```python
from build123d import *

# Parameters (mm, degrees)
SKETCH2_W               = 150
SKETCH2_H               = 180
BOSS_EXTRUDE1_DEPTH     = 4
SKETCH3_R               = 2
SKETCH3_W               = 23
SKETCH3_H               = 42
CUT_EXTRUDE1_DEPTH      = 118.426572802
MIRROR2_COPY_1_SKETCH_R = 2
MIRROR2_COPY_1_SKETCH_W = 23
MIRROR2_COPY_1_SKETCH_H = 42
MIRROR2_COPY_1_DEPTH    = 118.426572802
FILLET1_SIZE            = 10
FILLET1_SIZE_2          = 20
FILLET2_SIZE            = 10
FILLET2_SIZE_2          = 20
SKETCH4_W               = 50
SKETCH4_H               = 100
CUT_EXTRUDE2_DEPTH      = 118.426572949
SKETCH5_R               = 2.5
CUT_EXTRUDE3_DEPTH      = 118.426572949
SKETCH6_R               = 2.5
CUT_EXTRUDE4_DEPTH      = 118.426572949


with BuildPart() as part:
    # Sketch2 → Boss-Extrude1 (new, symmetric)
    with BuildSketch(Plane(origin=(0, 0, 0), x_dir=(1, 0, 0), z_dir=(0, 1, 0))):
        Rectangle(SKETCH2_W, SKETCH2_H)
    extrude(amount=BOSS_EXTRUDE1_DEPTH, both=True)

    # Sketch3 → Cut-Extrude1 (cut, through all)
    with BuildSketch(Plane(origin=(0, 4, 0), x_dir=(1, 0, 0), z_dir=(0, 1, 0))):
        with Locations(Location((-59.95, -34.7, 0), (0, 0, 270))):
            Circle(SKETCH3_R)
        with Locations(Location((-50.05, -34.7, 0), (0, 0, 270))):
            Circle(SKETCH3_R)
        with Locations(Location((-59.95, -83.3, 0), (0, 0, 270))):
            Circle(SKETCH3_R)
        with Locations(Location((-50.05, -83.3, 0), (0, 0, 270))):
            Circle(SKETCH3_R)
        with Locations((-55, -59)):
            Rectangle(SKETCH3_W, SKETCH3_H)
    cut_extrude1 = extrude(amount=-CUT_EXTRUDE1_DEPTH, mode=Mode.SUBTRACT)

    # Mirror1: Cut-Extrude1 across plane
    add(cut_extrude1.mirror(Plane.XY), mode=Mode.SUBTRACT)

    # Mirror2: Cut-Extrude1 across plane
    add(cut_extrude1.mirror(Plane(origin=(0, 0, 0), x_dir=(0, 0, 1), z_dir=(1, 0, 0))), mode=Mode.SUBTRACT)

    # Mirror2 copy 1 sketch → Mirror2 copy 1 (cut, through all)
    with BuildSketch(Plane(origin=(0, 4, 0), x_dir=(-1, 0, 0), z_dir=(0, 1, 0))):
        with Locations(Location((-59.95, -34.7, 0), (0, 0, 270))):
            Circle(MIRROR2_COPY_1_SKETCH_R)
        with Locations(Location((-50.05, -34.7, 0), (0, 0, 270))):
            Circle(MIRROR2_COPY_1_SKETCH_R)
        with Locations(Location((-59.95, -83.3, 0), (0, 0, 270))):
            Circle(MIRROR2_COPY_1_SKETCH_R)
        with Locations(Location((-50.05, -83.3, 0), (0, 0, 270))):
            Circle(MIRROR2_COPY_1_SKETCH_R)
        with Locations((-55, -59)):
            Rectangle(MIRROR2_COPY_1_SKETCH_W, MIRROR2_COPY_1_SKETCH_H)
    extrude(amount=-MIRROR2_COPY_1_DEPTH, mode=Mode.SUBTRACT)

    # Fillet1
    # an asymmetric fillet: 20, 10 mm, written as the material it takes off along each edge
    with BuildSketch(Plane(origin=(-75, -54, -90), x_dir=(1, 0, 0), z_dir=(0, 1, 0))) as fillet1_piece_1:
        with BuildLine():
            Bezier((FILLET1_SIZE, 0), (0, 0), (0, -FILLET1_SIZE_2), weights=[1, 0.707106781, 1])
            Line((0, -FILLET1_SIZE_2), (0, 0))
            Line((0, 0), (FILLET1_SIZE, 0))
        make_face()
    extrude(amount=108, mode=Mode.SUBTRACT)
    with BuildSketch(Plane(origin=(75, 54, 90), x_dir=(0, 0, -1), z_dir=(0, -1, 0))) as fillet1_piece_2:
        with BuildLine():
            Bezier((FILLET1_SIZE_2, 0), (0, 0), (0, -FILLET1_SIZE), weights=[1, 0.707106781, 1])
            Line((0, -FILLET1_SIZE), (0, 0))
            Line((0, 0), (FILLET1_SIZE_2, 0))
        make_face()
    extrude(amount=108, mode=Mode.SUBTRACT)

    # Fillet2
    # an asymmetric fillet: 20, 10 mm, written as the material it takes off along each edge
    with BuildSketch(Plane(origin=(75, 54, -90), x_dir=(-1, 0, 0), z_dir=(0, -1, 0))) as fillet2_piece_1:
        with BuildLine():
            Bezier((FILLET2_SIZE, 0), (0, 0), (0, -FILLET2_SIZE_2), weights=[1, 0.707106781, 1])
            Line((0, -FILLET2_SIZE_2), (0, 0))
            Line((0, 0), (FILLET2_SIZE, 0))
        make_face()
    extrude(amount=108, mode=Mode.SUBTRACT)
    with BuildSketch(Plane(origin=(-75, -54, 90), x_dir=(0, 0, -1), z_dir=(0, 1, 0))) as fillet2_piece_2:
        with BuildLine():
            Bezier((FILLET2_SIZE_2, 0), (0, 0), (0, -FILLET2_SIZE), weights=[1, 0.707106781, 1])
            Line((0, -FILLET2_SIZE), (0, 0))
            Line((0, 0), (FILLET2_SIZE_2, 0))
        make_face()
    extrude(amount=108, mode=Mode.SUBTRACT)

    # Sketch4 → Cut-Extrude2 (cut, through all)
    with BuildSketch(Plane(origin=(0, 4, 0), x_dir=(1, 0, 0), z_dir=(0, 1, 0))):
        Rectangle(SKETCH4_W, SKETCH4_H)
    extrude(amount=-CUT_EXTRUDE2_DEPTH, mode=Mode.SUBTRACT)

    # Sketch5 → Cut-Extrude3 (cut, through all)
    with BuildSketch(Plane(origin=(0, 4, 0), x_dir=(1, 0, 0), z_dir=(0, 1, 0))):
        with Locations(Location((-25, 81, 0), (0, 0, 270))):
            Circle(SKETCH5_R)
        with Locations(Location((25, 81, 0), (0, 0, 270))):
            Circle(SKETCH5_R)
        with Locations(Location((0, 81, 0), (0, 0, 270))):
            Circle(SKETCH5_R)
        with Locations(Location((-25, 70, 0), (0, 0, 270))):
            Circle(SKETCH5_R)
        with Locations(Location((0, 70, 0), (0, 0, 270))):
            Circle(SKETCH5_R)
        with Locations(Location((25, 70, 0), (0, 0, 270))):
            Circle(SKETCH5_R)
        with Locations(Location((-25, 59, 0), (0, 0, 270))):
            Circle(SKETCH5_R)
        with Locations(Location((0, 59, 0), (0, 0, 270))):
            Circle(SKETCH5_R)
        with Locations(Location((25, 59, 0), (0, 0, 270))):
            Circle(SKETCH5_R)
    cut_extrude3 = extrude(amount=-CUT_EXTRUDE3_DEPTH, mode=Mode.SUBTRACT)

    # Sketch6 → Cut-Extrude4 (cut, through all)
    with BuildSketch(Plane(origin=(0, 4, 0), x_dir=(1, 0, 0), z_dir=(0, 1, 0))):
        with Locations(Location((-67, 17.5, 0), (0, 0, 270))):
            Circle(SKETCH6_R)
        with Locations(Location((-67, -17.5, 0), (0, 0, 270))):
            Circle(SKETCH6_R)
        with Locations(Location((-67, 0, 0), (0, 0, 270))):
            Circle(SKETCH6_R)
        with Locations(Location((-52, 0, 0), (0, 0, 270))):
            Circle(SKETCH6_R)
        with Locations(Location((-52, 17.5, 0), (0, 0, 270))):
            Circle(SKETCH6_R)
        with Locations(Location((-52, -17.5, 0), (0, 0, 270))):
            Circle(SKETCH6_R)
        with Locations(Location((-37, 0, 0), (0, 0, 270))):
            Circle(SKETCH6_R)
        with Locations(Location((-37, 17.5, 0), (0, 0, 270))):
            Circle(SKETCH6_R)
        with Locations(Location((-37, -17.5, 0), (0, 0, 270))):
            Circle(SKETCH6_R)
    cut_extrude4 = extrude(amount=-CUT_EXTRUDE4_DEPTH, mode=Mode.SUBTRACT)

    # Mirror4: Cut-Extrude4 across plane
    add(cut_extrude4.mirror(Plane(origin=(0, 0, 0), x_dir=(0, 0, 1), z_dir=(1, 0, 0))), mode=Mode.SUBTRACT)

    # Mirror5: Cut-Extrude3 across plane
    add(cut_extrude3.mirror(Plane.XY), mode=Mode.SUBTRACT)


solid = part.part
```
Check sheet for the modelled part. Datum: model origin and axes. Units: mm. Round coordinates to 2 decimals unless told otherwise and drop trailing zeros. Order: outer loops, then holes, each group sorted by start corner. A loop starts at its lowest first (then second) coordinate and runs counter-clockwise, first axis right, second up. Notation, with made-up numbers: (85, 51) - (138, 51) arc R24 cw to (138, 63) - close; hole circle Ø6 at (76.5, -4). An arc over 180 degrees is marked (long way). Answer as CSV lines item,"result". Start each with the question number.
1) Section check D-D (z = -17.5). Give the number of separate pieces and of enclosed holes in the cut face, then the cut area to 3 significant figures.
2) Section check A-A (x = -16). Record the cut outline in (y, z).
3) Section check C-C (z = 34.7). Record the cut outline in (x, y).
4) Section check B-B (x = -37). Record the cut outline in (y, z).
5) Draft check along Z on faces 1 (the face through (50, 0.1, 81.3)), 2 (the face through (-34, -4, -1)). Enter one of: +Z half, -Z half, draft (parallel to the pull), parting line (faces both ways), or undercut.
6) Scan lines: probe 1 along Z at (x, y) = (55.5, -2.25); probe 2 along X at (y, z) = (-2.75, 44); probe 3 along X at (y, z) = (-0.5, 59). Record each from-to range of solid material in increasing order.
Determined:
1,separate pieces,"8"
1,enclosed holes,"0"
1,area,"560 mm^2"
2,outline,"(-4, -90) - (4, -90) - (4, -50) - (-4, -50) - close; (-4, 50) - (4, 50) - (4, 90) - (-4, 90) - close"
3,outline,"(-75, -4) - (-61.95, -4) - (-61.95, 4) - (-75, 4) - close; (-57.95, -4) - (-52.05, -4) - (-52.05, 4) - (-57.95, 4) - close; (-48.05, -4) - (-25, -4) - (-25, 4) - (-48.05, 4) - close; (25, -4) - (48.05, -4) - (48.05, 4) - (25, 4) - close; (52.05, -4) - (57.95, -4) - (57.95, 4) - (52.05, 4) - close; (61.95, -4) - (75, -4) - (75, 4) - (61.95, 4) - close"
4,outline,"(-4, -90) - (4, -90) - (4, -20) - (-4, -20) - close; (-4, -15) - (4, -15) - (4, -2.5) - (-4, -2.5) - close; (-4, 2.5) - (4, 2.5) - (4, 15) - (-4, 15) - close; (-4, 20) - (4, 20) - (4, 90) - (-4, 90) - close"
5,face 1,"undercut"
5,face 2,"draft"
6,probe 1,"-90 to -80, -38 to 38, 80 to 90"
6,probe 2,"-75 to -66.5, -43.5 to -25, 25 to 43.5, 66.5 to 75"
6,probe 3,"-75 to -66.5, -43.5 to -27.5, -22.5 to -2.5, 2.5 to 22.5, 27.5 to 43.5, 66.5 to 75"
